Work out the finished part from the listing and answer in its coordinate system (mm). Round coordinates to 2 decimals unless told otherwise and drop trailing zeros. Write each loop counter-clockwise with the first axis right and the second up, starting at its lowest first coordinate (ties: lowest second). Pieces come first, ordered by that corner, then holes.
1. Find section A-A (z = -41.75). Write down the section's boundary in (x, y).
2. Find section D-D (x = -11.5). Write down the section's boundary in (y, z), and give its area (3 significant figures).
3. Straight lines are drawn through the part: probe 1 along Z at (x, y) = (2.5, 3.3); probe 2 along X at (y, z) = (2.3, -25); probe 3 along X at (y, z) = (3, -7.5). For each, find the intervals that lie inside material, in ascending order.
4. Find section B-B (x = 0). Write down the section's boundary in (y, z).
5. Flat-ended cylindrical pins translate along their axes: pin 1 Ø1 at (y, z) = (3, -11.5) entering from +X; pin 2 Ø2.5 at (y, z) = (3, -5) entering from +X; pin 3 Ø3 at (y, z) = (3.5, -24.5) entering from +X. Find the tip coordinate at first contact, or state that the pin passes through.
6. Find section C-C (y = 1.25). Count the separate pieces of the cut face and the enclosed holes in it, and give its area (3 significant figures).
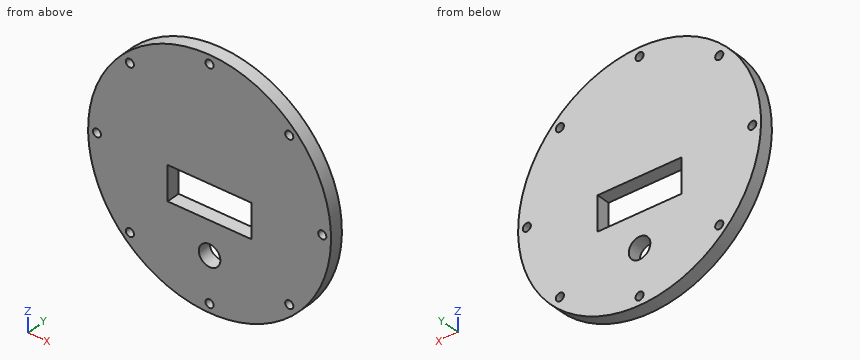
```python
from build123d import *

# Parameters (mm, degrees)
SKETCH1_R           = 45
SKETCH1_R_2         = 1.5
BOSS_EXTRUDE2_DEPTH = 5
SKETCH2_W           = 31
SKETCH2_H           = 12.7
CUT_EXTRUDE2_DEPTH  = 10
SKETCH4_R           = 4
CUT_EXTRUDE6_DEPTH  = 10


with BuildPart() as part:
    # Sketch1 → Boss-Extrude2 (new body)
    with BuildSketch(Plane(origin=(0, 0, 0), x_dir=(1, 0, 0), z_dir=(0, 1, 0))):
        with Locations(Location((0, 0, 0), (0, 0, 270))):
            Circle(SKETCH1_R)
        with Locations(Location((0, 41.75, 0), (0, 0, 270))):
            Circle(SKETCH1_R_2, mode=Mode.SUBTRACT)
        with Locations(Location((29.521708115, 29.521708115, 0), (0, 0, 270))):
            Circle(SKETCH1_R_2, mode=Mode.SUBTRACT)
        with Locations(Location((41.75, 0, 0), (0, 0, 270))):
            Circle(SKETCH1_R_2, mode=Mode.SUBTRACT)
        with Locations(Location((29.521708115, -29.521708115, 0), (0, 0, 270))):
            Circle(SKETCH1_R_2, mode=Mode.SUBTRACT)
        with Locations(Location((0, -41.75, 0), (0, 0, 270))):
            Circle(SKETCH1_R_2, mode=Mode.SUBTRACT)
        with Locations(Location((-29.521708115, -29.521708115, 0), (0, 0, 270))):
            Circle(SKETCH1_R_2, mode=Mode.SUBTRACT)
        with Locations(Location((-41.75, 0, 0), (0, 0, 270))):
            Circle(SKETCH1_R_2, mode=Mode.SUBTRACT)
        with Locations(Location((-29.521708115, 29.521708115, 0), (0, 0, 270))):
            Circle(SKETCH1_R_2, mode=Mode.SUBTRACT)
    extrude(amount=BOSS_EXTRUDE2_DEPTH)

    # Sketch2 → Cut-Extrude2 (cut)
    with BuildSketch(Plane(origin=(0, 5, 0), x_dir=(1, 0, 0), z_dir=(0, 1, 0))):
        with Locations((0, 6.35)):
            Rectangle(SKETCH2_W, SKETCH2_H)
    extrude(amount=-CUT_EXTRUDE2_DEPTH, mode=Mode.SUBTRACT)

    # Sketch4 → Cut-Extrude6 (cut)
    with BuildSketch(Plane(origin=(0, 5, 0), x_dir=(1, 0, 0), z_dir=(0, 1, 0))):
        with Locations(Location((0, 25, 0), (0, 0, 270))):
            Circle(SKETCH4_R)
    extrude(amount=-CUT_EXTRUDE6_DEPTH, mode=Mode.SUBTRACT)


solid = part.part
```
Worked answers:
1. outline: (-16.79, 0) - (-1.5, 0) - (-1.5, 5) - (-16.79, 5) - close; (1.5, 0) - (16.79, 0) - (16.79, 5) - (1.5, 5) - close
2. outline: (0, -43.51) - (5, -43.51) - (5, -12.7) - (0, -12.7) - close; (0, 0) - (5, 0) - (5, 43.51) - (0, 43.51) - close
2. area: 372 mm2
3. probe 1: z = -44.93 to -28.12, -21.88 to -12.7, 0 to 44.93
3. probe 2: x = -37.42 to -4, 4 to 37.42
3. probe 3: x = -44.37 to -15.5, 15.5 to 44.37
4. outline: (0, -45) - (5, -45) - (5, -43.25) - (0, -43.25) - close; (0, -40.25) - (5, -40.25) - (5, -29) - (0, -29) - close; (0, -21) - (5, -21) - (5, -12.7) - (0, -12.7) - close; (0, 0) - (5, 0) - (5, 40.25) - (0, 40.25) - close; (0, 43.25) - (5, 43.25) - (5, 45) - (0, 45) - close
5. pin 1: stops at x = 43.63
5. pin 2: stops at x = 44.84
5. pin 3: stops at x = 38.68
6. separate pieces: 1
6. enclosed holes: 10
6. area: 5,860 mm2
